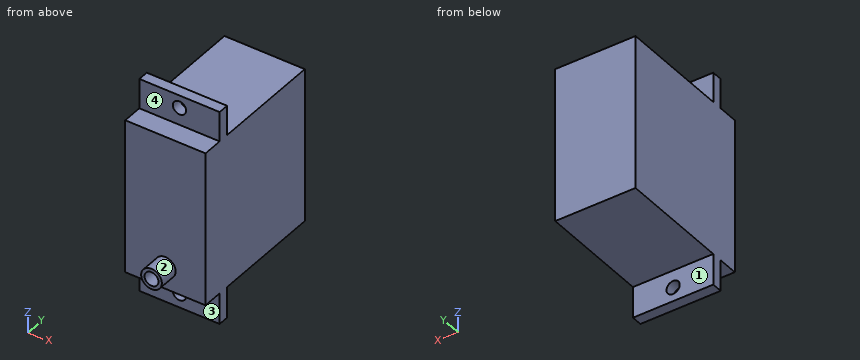
from build123d import *

# Parameters (mm, degrees)
SKETCH_3_W          = 32.5
SKETCH_3_H          = 21.45
EXTRUDE_1_DEPTH     = 6.05
CUT_EXTRUDE_START   = -3.86581
SKETCH_4_W          = 12.1
SKETCH_4_H          = 4.7
SKETCH_4_H_2        = 4.6
CUT_EXTRUDE_1_DEPTH = 26.951221363
CUT_EXTRUDE_START_2 = -5.46581
SKETCH_4_2_W        = 12.1
SKETCH_4_2_H        = 4.7
SKETCH_4_2_H_2      = 4.6
CUT_EXTRUDE_2_DEPTH = 17.619601363
SKETCH_5_R          = 1
CUT_EXTRUDE_3_DEPTH = 23.085411363
SKETCH_7_R          = 1.557821419
SKETCH_7_R_2        = 1.04903278
EXTRUDE_3_DEPTH     = 3


with BuildPart() as part:
    # Sketch 3 → Extrude 1 (new, symmetric)
    with BuildSketch(Plane(origin=(0, 0, 0), x_dir=(0, 0, -1), z_dir=(1, 0, 0))):
        with Locations((-0.5985, 2.2091)):
            Rectangle(SKETCH_3_W, SKETCH_3_H)
    extrude(amount=EXTRUDE_1_DEPTH, both=True)

    # Sketch 4 → Cut-Extrude 1 (cut, through all)
    with BuildSketch(Plane(origin=(0, 0, 0), x_dir=(1, 0, 0), z_dir=(0, 1, 0)).offset(CUT_EXTRUDE_START)):
        with Locations((0, 13.30155)):
            Rectangle(SKETCH_4_W, SKETCH_4_H)
        with Locations((0, -14.6484)):
            Rectangle(SKETCH_4_W, SKETCH_4_H_2)
    extrude(amount=CUT_EXTRUDE_1_DEPTH, mode=Mode.SUBTRACT)

    # Sketch 4_2 → Cut-Extrude 2 (cut, through all)
    with BuildSketch(Plane(origin=(0, 0, 0), x_dir=(1, 0, 0), z_dir=(0, 1, 0)).offset(CUT_EXTRUDE_START_2)):
        with Locations((0, 13.30155)):
            Rectangle(SKETCH_4_2_W, SKETCH_4_2_H)
        with Locations((0, -14.6484)):
            Rectangle(SKETCH_4_2_W, SKETCH_4_2_H_2)
    extrude(amount=-CUT_EXTRUDE_2_DEPTH, mode=Mode.SUBTRACT)

    # Sketch 5 → Cut-Extrude 3 (cut, through all)
    with BuildSketch(Plane(origin=(0, 0, 0), x_dir=(1, 0, 0), z_dir=(0, 1, 0))):
        with Locations(Location((0, 13.55, 0), (0, 0, 90))):
            Circle(SKETCH_5_R)
        with Locations(Location((0, -14.949238683, 0), (0, 0, 90))):
            Circle(SKETCH_5_R)
    extrude(amount=-CUT_EXTRUDE_3_DEPTH, mode=Mode.SUBTRACT)

    # Sketch 7 → Extrude 3 (add)
    with BuildSketch(Plane.XZ.offset(8.5159)):
        with Locations(Location((0, -7.64347992, 0), (0, 0, 90))):
            Circle(SKETCH_7_R)
        with Locations(Location((0, -7.64347992, 0), (0, 0, 270))):
            Circle(SKETCH_7_R_2, mode=Mode.SUBTRACT)
    extrude(amount=EXTRUDE_3_DEPTH)


solid = part.part
Verification items for the finished model (mm, model axes). Face numbers are marked on the shaded views. A direction names the side the tool comes from. Coordinates: 2 decimals unless noted, no trailing zeros. Order: outer loops, then holes, each group sorted by start corner. A loop starts at its lowest first (then second) coordinate and runs counter-clockwise, first axis right, second up.
1. Set-up check for the marked faces 1, 2, 3 and 4: record each of +Z, -Z, +X, -X, +Y, -Y from which the full face is reachable in a straight line by a thin tool's end or side.
Results found:
face 1: -Z, +X, -X, +Y
face 2: -Y
face 3: -Z, +X, -X, -Y
face 4: +Z, +X, -X, -Y
2. Sectioned sample at A-A, the plane z = 14.5. Record the cut outline in (x, y).
Results found:
outline: (-6.05, -5.47) - (-0.89, -5.47) - (-0.89, -3.87) - (-6.05, -3.87) - close; (0.89, -5.47) - (6.05, -5.47) - (6.05, -3.87) - (0.89, -3.87) - close
3. Sectioned sample at D-D, the plane z = -13.55. Record the cut outline in (x, y), and give its area (3 significant figures).
Results found:
outline: (-6.05, -5.47) - (-1, -5.47) - (-1, -3.87) - (-6.05, -3.87) - close; (1, -5.47) - (6.05, -5.47) - (6.05, -3.87) - (1, -3.87) - close
area: 16.2 mm2
4. Scan lines: line 1 (Y direction, x = -2.5, z = 4.5); line 2 (Z direction, x = -0.75, y = 1.25); line 3 (Y direction, x = -2, z = 13). Record each from-to range of solid material in increasing order.
Results found:
line 1: y = -8.52 to 12.93
line 2: z = -10.95 to 12.35
line 3: y = -5.47 to -3.87
5. Go/stop test with flat-tipped pins: pin 1 Ø1.5 at (x, y) = (-4, 0.5) entering from -Z; pin 2 Ø1.6 at (x, z) = (0, -13.55) entering from -Y; pin 3 Ø3 at (y, z) = (5, -12) entering from -X; pin 4 Ø1.4 at (x, z) = (-2.5, -13.5) entering from -Y. Record where each tip stops, or that it passes through.
Results found:
pin 1: stops at z = -10.95
pin 2: passes through
pin 3: stops at x = -6.05
pin 4: stops at y = -5.47
6. Sectioned sample at B-B, the plane x = 0. Record the cut outline in (y, z).
Results found:
outline: (-11.52, -9.2) - (-8.52, -9.2) - (-8.52, -10.95) - (-5.47, -10.95) - (-5.47, -12.55) - (-3.87, -12.55) - (-3.87, -10.95) - (12.93, -10.95) - (12.93, 12.35) - (-3.87, 12.35) - (-3.87, 13.95) - (-5.47, 13.95) - (-5.47, 12.35) - (-8.52, 12.35) - (-8.52, -6.09) - (-11.52, -6.09) - (-11.52, -6.59) - (-8.52, -6.59) - (-8.52, -8.69) - (-11.52, -8.69) - close; (-5.47, -15.65) - (-3.87, -15.65) - (-3.87, -14.55) - (-5.47, -14.55) - close; (-5.47, 15.95) - (-3.87, 15.95) - (-3.87, 16.85) - (-5.47, 16.85) - close
7. Sectioned sample at C-C, the plane x = -3. Record the cut outline in (y, z), and give its area (3 significant figures).
Results found:
outline: (-8.52, -10.95) - (-5.47, -10.95) - (-5.47, -15.65) - (-3.87, -15.65) - (-3.87, -10.95) - (12.93, -10.95) - (12.93, 12.35) - (-3.87, 12.35) - (-3.87, 16.85) - (-5.47, 16.85) - (-5.47, 12.35) - (-8.52, 12.35) - close
area: 515 mm2
